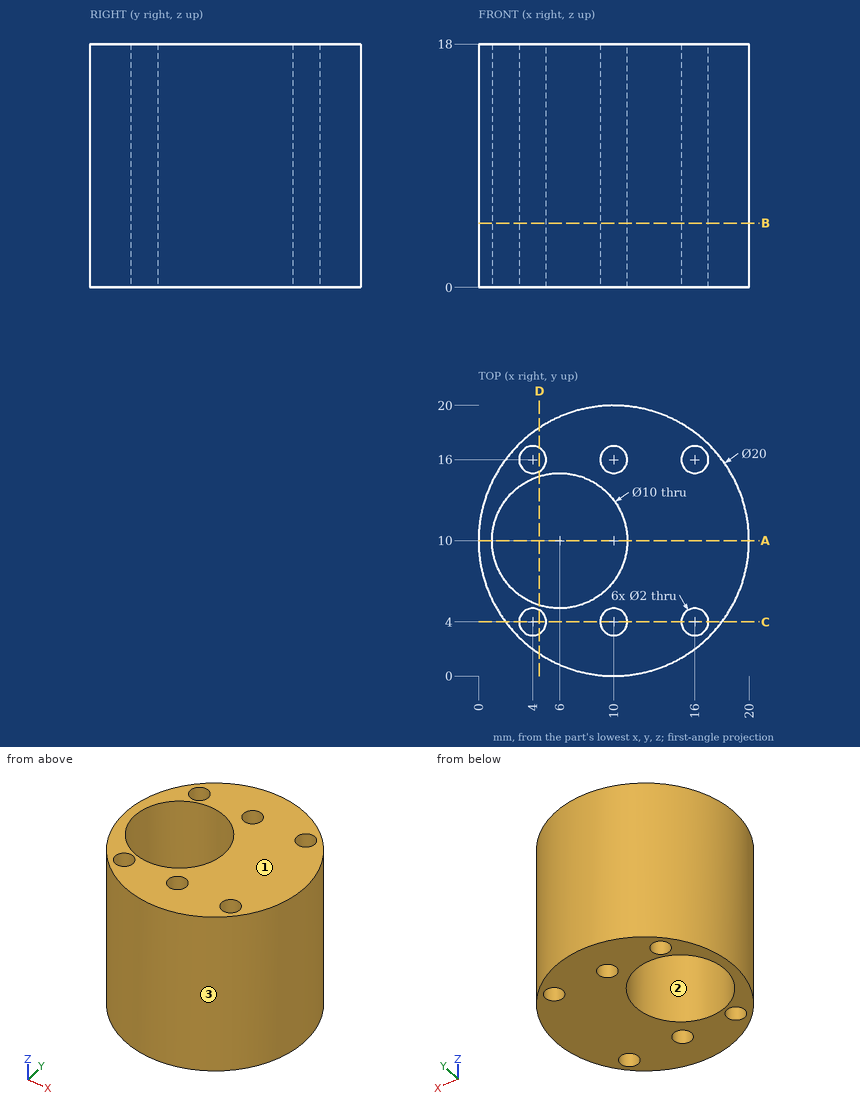
Design review of the part shown in the three views and the two pictorial views. Dimensions are in mm from the part's minimum x, y and z. Give positions to 0.01 mm unless a question says otherwise; leave off trailing zeros. Loops run counter-clockwise (first coordinate to the right, second up) from the corner with the lowest first, then second, coordinate; pieces in that order, holes last. Notation, with made-up numbers: (3, -17.5) -> (61, -17.5) arc R15 cw to (61, -13.5) -> close; hole circle Ø3 at (79.5, 82). An arc over 180 degrees is marked (long way). Answer as a JSON object with one key per item and string values. Group by question number.
Q1. Take a section at D-D (x = 4.5). Write out the cut boundary in (y, z), plus the area to 3 significant figures.
Q2. Take a section at C-C (y = 4). Write out the cut boundary in (x, z), plus the area to 3 significant figures.
Q3. Take a section at A-A (y = 10). Write out the cut boundary in (x, z).
Q4. Insertion check: pin 1 (10 mm diameter, centred on y = 17.5, z = 6, fed in from +X); pin 2 (1.8 mm diameter, centred on x = 16, y = 4, fed in from +Z); pin 3 (1 mm diameter, centred on x = 15.5, z = 9, fed in from -Y); pin 4 (4 mm diameter, centred on x = 16.5, z = 10, fed in from -Y). Each pin has a flat end and moves straight along its axis. Give the tip position at first contact, or say it passes through.
Q5. Take a section at B-B (z = 4.75). Write out the cut boundary in (x, y), plus the area to 3 significant figures.
Q6. Draft analysis for pull direction Y (two halves, no side actions). For the marked faces 1, 2 and 3, state which applies: pulls with the +Y half, pulls with the -Y half, needs draft (parallel to the pull), parting line crosses it, or undercut.
Q7. Wall thickness on line 1 along Y through (x, z) = (4, 14); line 2 along Y through (x, z) = (10, 4); line 3 along Y through (x, z) = (16, 6.75): over which ranges is each line inside the solid? List them lowest first.
Answer below:
{
 "1": {"outline": "(1.65, 0) -> (3.13, 0) -> (3.13, 18) -> (1.65, 18) -> close; (4.87, 0) -> (5.23, 0) -> (5.23, 18) -> (4.87, 18) -> close; (14.77, 0) -> (15.13, 0) -> (15.13, 18) -> (14.77, 18) -> close; (16.87, 0) -> (18.35, 0) -> (18.35, 18) -> (16.87, 18) -> close", "area": "66.6 mm2"},
 "2": {"outline": "(2, 0) -> (3, 0) -> (3, 18) -> (2, 18) -> close; (5, 0) -> (9, 0) -> (9, 18) -> (5, 18) -> close; (11, 0) -> (15, 0) -> (15, 18) -> (11, 18) -> close; (17, 0) -> (18, 0) -> (18, 18) -> (17, 18) -> close", "area": "180 mm2"},
 "3": {"outline": "(0, 0) -> (1, 0) -> (1, 18) -> (0, 18) -> close; (11, 0) -> (20, 0) -> (20, 18) -> (11, 18) -> close"},
 "4": {"pin 1": "stops at x = 19.68", "pin 2": "passes through", "pin 3": "stops at y = 1.34", "pin 4": "stops at y = 1.07"},
 "5": {"outline": "circle Ø20 at (10, 10); hole circle Ø10 at (6, 10); hole circle Ø2 at (4, 4); hole circle Ø2 at (4, 16); hole circle Ø2 at (10, 4); hole circle Ø2 at (10, 16); hole circle Ø2 at (16, 4); hole circle Ø2 at (16, 16)", "area": "217 mm2"},
 "6": {"face 1": "needs draft", "face 2": "undercut", "face 3": "parting line crosses it"},
 "7": {"line 1": "y = 2 to 3, 5 to 5.42, 14.58 to 15, 17 to 18", "line 2": "y = 0 to 3, 5 to 7, 13 to 15, 17 to 20", "line 3": "y = 2 to 3, 5 to 15, 17 to 18"}
}
